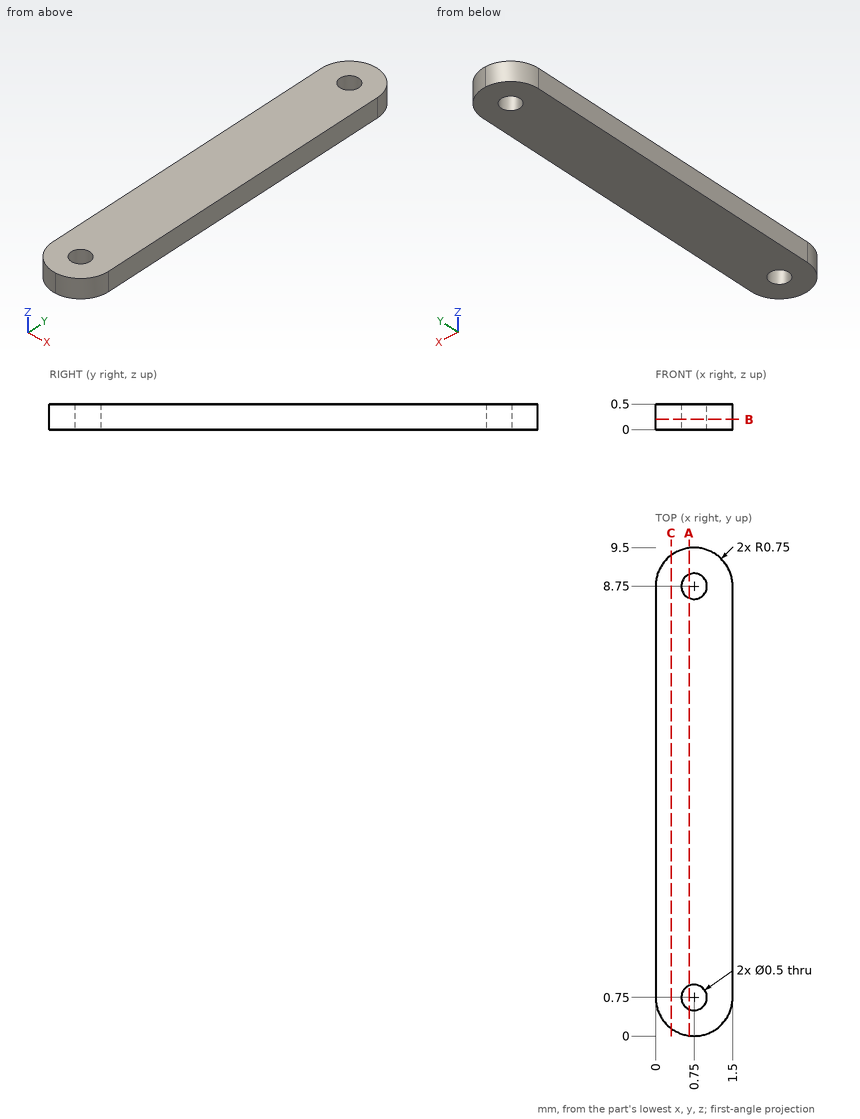
The drawing under review shows one solid part. Ordinate dimensions are in mm from its lowest x, y, z. Give positions to 0.01 mm unless a question says otherwise; leave off trailing zeros. Order: outer loops, then holes, each group sorted by start corner. A loop starts at its lowest first (then second) coordinate and runs counter-clockwise, first axis right, second up. Notation, with made-up numbers: M -25,37 L 7,37 A28 ccw 7,72 Z; hole C 68.5,15.25 d10. An arc over 180 degrees is marked long. Answer in a Markdown table with one row per item. Add a question column.
1. To check wall thickness, follow line 1 along Y through (x, z) = (0.7, 0.2); line 2 along X through (y, z) = (8.75, 0.35); line 3 along Y through (x, z) = (0.9, 0.25). State the ranges of each line that lie inside material, in increasing order.
2. Add section B-B on z = 0.2. State the section outline as (x, y) points.
3. Add section A-A on x = 0.65. State the section outline as (y, z) points, plus the area to 3 significant figures.
4. Add section C-C on x = 0.3. State the section outline as (y, z) points.
The answers:
| question | item | result |
|---|---|---|
| 1 | line 1 | 0 to 0.51, 0.99 to 8.51, 8.99 to 9.5 |
| 1 | line 2 | 0 to 0.5, 1 to 1.5 |
| 1 | line 3 | 0.02 to 0.55, 0.95 to 8.55, 8.95 to 9.48 |
| 2 | outline | M 0,0.75 A0.75 ccw 1.5,0.75 L 1.5,8.75 A0.75 ccw 0,8.75 Z; hole C 0.75,0.75 d0.5; hole C 0.75,8.75 d0.5 |
| 3 | outline | M 0.01,0 L 0.52,0 L 0.52,0.5 L 0.01,0.5 Z; M 0.98,0 L 8.52,0 L 8.52,0.5 L 0.98,0.5 Z; M 8.98,0 L 9.49,0 L 9.49,0.5 L 8.98,0.5 Z |
| 3 | area | 4.29 mm2 |
| 4 | outline | M 0.15,0 L 9.35,0 L 9.35,0.5 L 0.15,0.5 Z |
